The drawing under review shows one solid part. Ordinate dimensions are in mm from its lowest x, y, z. A direction names the side the tool comes from. Coordinates: 2 decimals unless noted, no trailing zeros. Write each loop counter-clockwise with the first axis right and the second up, starting at its lowest first coordinate (ties: lowest second). Pieces come first, ordered by that corner, then holes. Notation, with made-up numbers: (66, -9.75) -> (108, -9.75) arc R36 cw to (108, 26.25) -> close; hole circle Ø8 at (21, -14.75). An arc over 180 degrees is marked (long way). One line per question, with ' | ' between items. Start each with the question number.
Q1. Add section C-C on x = 4. State the section outline as (y, z) points.
Q2. Wall thickness on probe 1 along Y at (x, z) = (12.5, 55.2); probe 2 along Y at (x, z) = (21, 55.3); probe 3 along X at (y, z) = (25.9, 26): over which ranges is each line inside the solid? List them lowest first.
Q3. Add section A-A on z = 36. State the section outline as (x, y) points.
Q4. For the marked faces 1 and 2, list the 3-axis set-ups (+Z, -Z, +X, -X, +Y, -Y) from which the entire face can be reached by the end or side of a thin tool; tool diameter is ignored.
Q5. For P1, Ø1.8, axis at x = 12.5, z = 6, coming from the -Y side; P2, Ø4, axis at x = 12.5, z = 46, coming from the +Y side; P3, Ø5, axis at x = 14, y = 12.5, coming from the -Z side; P4, Ø5, axis at x = 11, z = 13.5, coming from the -Y side, all flat-tipped, find the tip position at first contact; note any pin that passes through.
Q6. Add section B-B on y = 13.5. State the section outline as (x, z) points, and give its area (3 significant figures).
Q7. Add section D-D on y = 5. State the section outline as (x, z) points, and give its area (3 significant figures).
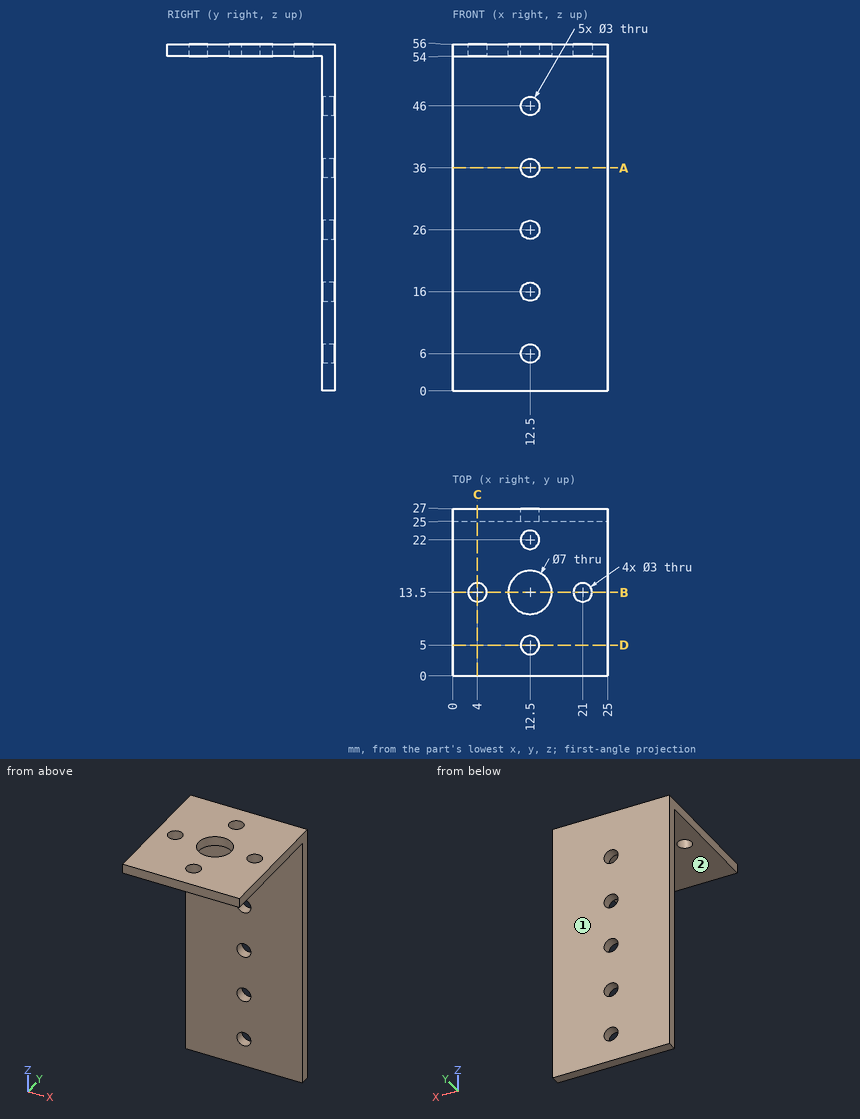
Output values:
1) outline: (0, 54) -> (12, 54) -> (12, 56) -> (0, 56) -> close; (15, 54) -> (25, 54) -> (25, 0) -> (27, 0) -> (27, 56) -> (15, 56) -> close
2) probe 1: y = 0 to 3.5, 6.5 to 10, 17 to 20.5, 23.5 to 27 | probe 2: y = 0 to 12, 15 to 27 | probe 3: x = 0 to 11, 14 to 25
3) outline: (0, 25) -> (11, 25) -> (11, 27) -> (0, 27) -> close; (14, 25) -> (25, 25) -> (25, 27) -> (14, 27) -> close
4) face 1: +Z, -Z, +X, -X, +Y | face 2: -Z, +X, -X, -Y
5) P1: passes through | P2: stops at y = 27 | P3: stops at z = 54 | P4: stops at y = 25
6) outline: (0, 54) -> (2.5, 54) -> (2.5, 56) -> (0, 56) -> close; (5.5, 54) -> (9, 54) -> (9, 56) -> (5.5, 56) -> close; (16, 54) -> (19.5, 54) -> (19.5, 56) -> (16, 56) -> close; (22.5, 54) -> (25, 54) -> (25, 56) -> (22.5, 56) -> close | area: 24.0 mm2
7) outline: (0, 54) -> (11, 54) -> (11, 56) -> (0, 56) -> close; (14, 54) -> (25, 54) -> (25, 56) -> (14, 56) -> close | area: 44.0 mm2
